from build123d import *

# Parameters (mm, degrees)
SKETCH1_W               = 38.1
SKETCH1_H               = 31.75
BOSS_EXTRUDE1_DEPTH     = 9.525
CUT_EXTRUDE2_DEPTH      = 4.2926
SKETCH3_R               = 2.0574
CUT_EXTRUDE3_DEPTH      = 8.89
SKETCH7_R               = 2.0574
CUT_EXTRUDE5_DEPTH      = 8.89
SKETCH8_R               = 0.889
CUT_EXTRUDE6_DEPTH      = 4.7625
MIRROR4_COPY_1_SKETCH_R = 0.889
MIRROR4_COPY_1_DEPTH    = 4.7625
SKETCH11_R              = 0.889
CUT_EXTRUDE7_DEPTH      = 4.7625
MIRROR6_COPY_1_SKETCH_R = 0.889
MIRROR6_COPY_1_DEPTH    = 4.7625
SKETCH12_R              = 0.889
CUT_EXTRUDE9_DEPTH      = 7.9375


with BuildPart() as part:
    # Sketch1 → Boss-Extrude1 (new body)
    with BuildSketch(Plane(origin=(0, 0, 0), x_dir=(1, 0, 0), z_dir=(0, 1, 0))):
        Rectangle(SKETCH1_W, SKETCH1_H)
    extrude(amount=BOSS_EXTRUDE1_DEPTH)

    # Sketch2 → Cut-Extrude2 (cut)
    with BuildSketch(Plane(origin=(0, 9.525, 0), x_dir=(1, 0, 0), z_dir=(0, 1, 0))):
        with BuildLine():
            Line((-11.90625, -9.525), (11.90625, -9.525))
            ThreePointArc((11.90625, -9.525), (12.467516008, -9.292516008), (12.7, -8.73125))
            Line((12.7, -8.73125), (12.7, 8.73125))
            ThreePointArc((12.7, 8.73125), (12.467516008, 9.292516008), (11.90625, 9.525))
            Line((11.90625, 9.525), (-11.90625, 9.525))
            ThreePointArc((-11.90625, 9.525), (-12.467516008, 9.292516008), (-12.7, 8.73125))
            Line((-12.7, 8.73125), (-12.7, -8.73125))
            ThreePointArc((-12.7, -8.73125), (-12.467516008, -9.292516008), (-11.90625, -9.525))
        make_face()
    extrude(amount=-CUT_EXTRUDE2_DEPTH, mode=Mode.SUBTRACT)

    # Sketch3 → Cut-Extrude3 (cut)
    with BuildSketch(Plane.ZY.offset(19.05)):
        with Locations((0, 5.2324)):
            Circle(SKETCH3_R)
    cut_extrude3 = extrude(amount=-CUT_EXTRUDE3_DEPTH, mode=Mode.SUBTRACT)

    # Mirror1: Cut-Extrude3 across plane
    add(cut_extrude3.mirror(Plane(origin=(0, 0, 0), x_dir=(0, 0, 1), z_dir=(1, 0, 0))), mode=Mode.SUBTRACT)

    # Sketch7 → Cut-Extrude5 (cut)
    with BuildSketch(Plane(origin=(0, 0, -15.875), x_dir=(-1, 0, 0), z_dir=(0, 0, -1))):
        with Locations((0, 5.2324)):
            Circle(SKETCH7_R)
    cut_extrude5 = extrude(amount=-CUT_EXTRUDE5_DEPTH, mode=Mode.SUBTRACT)

    # Mirror2: Cut-Extrude5 across plane
    add(cut_extrude5.mirror(Plane.XY), mode=Mode.SUBTRACT)

    # Sketch8 → Cut-Extrude6 (cut)
    with BuildSketch(Plane(origin=(19.05, 0, 0), x_dir=(0, 0, -1), z_dir=(1, 0, 0))):
        with Locations((6.6802, 5.2324)):
            Circle(SKETCH8_R)
    cut_extrude6 = extrude(amount=-CUT_EXTRUDE6_DEPTH, mode=Mode.SUBTRACT)

    # Mirror3: Cut-Extrude6 across plane
    add(cut_extrude6.mirror(Plane.XY), mode=Mode.SUBTRACT)

    # Mirror4: Cut-Extrude6 across plane
    add(cut_extrude6.mirror(Plane(origin=(0, 0, 0), x_dir=(0, 0, 1), z_dir=(1, 0, 0))), mode=Mode.SUBTRACT)

    # Mirror4 copy 1 sketch → Mirror4 copy 1 (cut)
    with BuildSketch(Plane.ZY.offset(19.05)):
        with Locations((6.6802, 5.2324)):
            Circle(MIRROR4_COPY_1_SKETCH_R)
    extrude(amount=-MIRROR4_COPY_1_DEPTH, mode=Mode.SUBTRACT)

    # Sketch11 → Cut-Extrude7 (cut)
    with BuildSketch(Plane.XY.offset(15.875)):
        with Locations((6.6802, 5.2324)):
            Circle(SKETCH11_R)
    cut_extrude7 = extrude(amount=-CUT_EXTRUDE7_DEPTH, mode=Mode.SUBTRACT)

    # Mirror5: Cut-Extrude7 across plane
    add(cut_extrude7.mirror(Plane(origin=(0, 0, 0), x_dir=(0, 0, 1), z_dir=(1, 0, 0))), mode=Mode.SUBTRACT)

    # Mirror6: Cut-Extrude7 across plane
    add(cut_extrude7.mirror(Plane.XY), mode=Mode.SUBTRACT)

    # Mirror6 copy 1 sketch → Mirror6 copy 1 (cut)
    with BuildSketch(Plane(origin=(0, 0, -15.875), x_dir=(-1, 0, 0), z_dir=(0, 0, -1))):
        with Locations((6.6802, 5.2324)):
            Circle(MIRROR6_COPY_1_SKETCH_R)
    extrude(amount=-MIRROR6_COPY_1_DEPTH, mode=Mode.SUBTRACT)

    # Sketch12 → Cut-Extrude9 (cut)
    with BuildSketch(Plane(origin=(0, 9.525, 0), x_dir=(1, 0, 0), z_dir=(0, 1, 0))):
        with Locations(Location((-15.53845, 12.36345, 0), (0, 0, 270))):
            Circle(SKETCH12_R)
        with Locations(Location((15.53845, 12.36345, 0), (0, 0, 270))):
            Circle(SKETCH12_R)
        with Locations(Location((-15.53845, -12.36345, 0), (0, 0, 270))):
            Circle(SKETCH12_R)
        with Locations(Location((15.53845, -12.36345, 0), (0, 0, 270))):
            Circle(SKETCH12_R)
    extrude(amount=-CUT_EXTRUDE9_DEPTH, mode=Mode.SUBTRACT)


solid = part.part
Work out the finished part from the listing and answer in its coordinate system (mm). A direction names the side the tool comes from. Coordinates: 2 decimals unless noted, no trailing zeros. Order: outer loops, then holes, each group sorted by start corner. A loop starts at its lowest first (then second) coordinate and runs counter-clockwise, first axis right, second up. Notation, with made-up numbers: (68.5, 87) - (125.5, 87) arc R12 cw to (125.5, 93) - close; hole circle Ø8 at (1, 54). An arc over 180 degrees is marked (long way). Put each result on its own line as item: value. Start each with the question number.
1) For a pull along Y with two mould halves and no side action, classify faces 6 (the cylindrical face through (0.446, 3.224, -12.48)), 7 (the flat face through (16, 1.588, -12)), 8 (the cylindrical face through (-14.657, 5.612, -12.479)) as released by +Y, released by -Y, zero draft, split by the parting line, or undercut.
2) For faces 1 (the flat face through (14.288, 5, -7)), 2 (the cylindrical face through (0.446, 3.224, 12.48)), 3 (the flat face through (-14.288, 5, -7)), 4 (the flat face through (0, 8, 9.525)), 5 (the flat face through (0, 4, 6.985)), determine the directions among +Z, -Z, +X, -X, +Y, -Y from which every point of the face is accessible in a straight line to the end or side of a thin tool.
3) Find section D-D (x = 8.5). Give the vertices of the cut face in (y, z) (3 decimals), plus the area to 3 significant figures.
4) Find section A-A (z = 14). Give the vertices of the cut face in (x, y) (3 decimals).
5) Find the intervals of material crossed by line 1 (X direction, y = 2, z = 12.5); line 2 (Z direction, x = 0, y = 7.5) (3 decimals); line 3 (X direction, y = 7, z = 4), in increasing order. Write a range as from..to.
6) Flat-ended cylindrical pins translate along their axes: pin 1 (0.5 mm diameter, centred on y = 5, z = -6.5, fed in from -X); pin 2 (1.5 mm diameter, centred on x = -3.5, z = -1.5, fed in from +Y); pin 3 (3.5 mm diameter, centred on x = 0, y = 5.23, fed in from +Z) (3 decimals). Find the tip coordinate at first contact, or state that the pin passes through.
7) Find section C-C (z = 0). Give the vertices of the cut face in (x, y) (3 decimals), plus the area to 3 significant figures.
8) Find section B-B (x = 0). Give the vertices of the cut face in (y, z) (3 decimals).
Results list:
1. face 6: undercut
1. face 7: released by +Y
1. face 8: zero draft
2. face 1: +X
2. face 2: +Z
2. face 3: -X
2. face 4: +Y
2. face 5: +Z, +Y
3. outline: (0, -15.875) - (9.525, -15.875) - (9.525, -9.525) - (5.232, -9.525) - (5.232, 9.525) - (9.525, 9.525) - (9.525, 15.875) - (0, 15.875) - close
3. area: 221 mm^2
4. outline: (-19.05, 0) - (19.05, 0) - (19.05, 9.525) - (-19.05, 9.525) - close; hole circle Ø1.778 at (-6.68, 5.232); hole circle Ø4.115 at (0, 5.232); hole circle Ø1.778 at (6.68, 5.232)
5. line 1: x = -19.05..-16.42, -14.66..14.66, 16.42..19.05
5. line 2: z = -15.875..-9.525, 9.525..15.875
5. line 3: x = -19.05..-12.7, 12.7..19.05
6. pin 1: stops at x = -14.29
6. pin 2: stops at y = 5.23
6. pin 3: stops at z = 6.985
7. outline: (-19.05, 0) - (19.05, 0) - (19.05, 3.175) - (10.16, 3.175) - (10.16, 5.232) - (-10.16, 5.232) - (-10.16, 3.175) - (-19.05, 3.175) - close; (-19.05, 7.29) - (-12.7, 7.29) - (-12.7, 9.525) - (-19.05, 9.525) - close; (12.7, 7.29) - (19.05, 7.29) - (19.05, 9.525) - (12.7, 9.525) - close
7. area: 191 mm^2
8. outline: (0, -15.875) - (3.175, -15.875) - (3.175, -6.985) - (5.232, -6.985) - (5.232, 6.985) - (3.175, 6.985) - (3.175, 15.875) - (0, 15.875) - close; (7.29, -15.875) - (9.525, -15.875) - (9.525, -9.525) - (7.29, -9.525) - close; (7.29, 9.525) - (9.525, 9.525) - (9.525, 15.875) - (7.29, 15.875) - close
